Verification items for the finished model (mm, model axes). A direction names the side the tool comes from. Round coordinates to 2 decimals unless told otherwise and drop trailing zeros. Order: outer loops, then holes, each group sorted by start corner. A loop starts at its lowest first (then second) coordinate and runs counter-clockwise, first axis right, second up.
```python
from build123d import *

# Parameters (mm, degrees)
SKETCH_1_R          = 1.95
EXTRUDE_1_DEPTH     = 3
SKETCH_2_R          = 1.45
SKETCH_2_W          = 20
SKETCH_2_H          = 40
CUT_EXTRUDE_1_DEPTH = 10
FILLET_1_R          = 1.5
FILLET_2_R          = 10
FILLET_3_R          = 2


with BuildPart() as part:
    # 草图1 → 凸台-拉伸1 (new body)
    with BuildSketch(Plane.XY):
        Polygon((0, 0), (0, 66), (38, 66), (38, 0), (25, -45.927575687), (25, -78.1), (13, -78.1), (13, -45.927575687), align=None)
        with Locations((4, 40)):
            Circle(SKETCH_1_R, mode=Mode.SUBTRACT)
        with Locations((34, 40)):
            Circle(SKETCH_1_R, mode=Mode.SUBTRACT)
        with Locations((4, 61)):
            Circle(SKETCH_1_R, mode=Mode.SUBTRACT)
        with Locations((34, 61)):
            Circle(SKETCH_1_R, mode=Mode.SUBTRACT)
        with Locations((19, -56.8)):
            Circle(SKETCH_1_R, mode=Mode.SUBTRACT)
        with Locations((19, -69.2)):
            Circle(SKETCH_1_R, mode=Mode.SUBTRACT)
    extrude(amount=EXTRUDE_1_DEPTH)

    # 草图2 → 切除-拉伸1 (cut)
    with BuildSketch(Plane.XY.offset(3)):
        with Locations((12, 15)):
            Circle(SKETCH_2_R)
        with Locations((26, 15)):
            Circle(SKETCH_2_R)
        Polygon((5, 10), (16, 10), (16, -38.16779197), (5, 0.694002842), align=None)
        with Locations((19, 40)):
            Rectangle(SKETCH_2_W, SKETCH_2_H)
        Polygon((22, 10), (22, -38.16779197), (33, 0.694002842), (33, 10), align=None)
    extrude(amount=-CUT_EXTRUDE_1_DEPTH, mode=Mode.SUBTRACT)

    # 圆角1
    fillet_1_edges = [part.edges().sort_by_distance(p)[0] for p in [
        (0, 0, 1.5),
        (38, 0, 1.5),
        (25, -78.1, 1.5),
        (13, -78.1, 1.5),
    ]]
    fillet(fillet_1_edges, radius=FILLET_1_R)

    # 圆角2
    fillet_2_edges = [part.edges().sort_by_distance(p)[0] for p in [
        (25, -45.927575687, 1.5),
        (13, -45.927575687, 1.5),
    ]]
    fillet(fillet_2_edges, radius=FILLET_2_R)

    # 圆角3
    fillet_3_edges = [part.edges().sort_by_distance(p)[0] for p in [
        (0, 66, 1.5),
        (38, 66, 1.5),
        (9, 20, 1.5),
        (9, 60, 1.5),
        (29, 60, 1.5),
        (29, 20, 1.5),
        (5, 0.694002842, 1.5),
        (5, 10, 1.5),
        (16, 10, 1.5),
        (16, -38.16779197, 1.5),
        (22, 10, 1.5),
        (33, 10, 1.5),
        (33, 0.694002842, 1.5),
        (22, -38.16779197, 1.5),
    ]]
    fillet(fillet_3_edges, radius=FILLET_3_R)


solid = part.part
```
1) Draft check along Z on faces 1 (the flat face through (19, -5, 0)), 2 (the flat face through (28, 10, 2)). Enter one of: released by +Z, released by -Z, zero draft, split by the parting line, or undercut.
2) Sectioned sample at A-A on y = 53.5. Record the cut outline in (x, z).
3) Sectioned sample at D-D on z = 0.8. Count the separate pieces of the cut face and the enclosed holes in it, then the cut area to 3 significant figures.
4) Scan lines: probe 1 along X at (y, z) = (0.5, 0.75); probe 2 along X at (y, z) = (43.5, 1); probe 3 along Y at (x, z) = (15, 1.65). Record each from-to range of solid material in increasing order.
5) Go/stop test with flat-tipped pins: pin 1 Ø1.5 at (y, z) = (-5, 1.5) entering from +X; pin 2 Ø2.5 at (x, y) = (4, 61) entering from -Z; pin 3 Ø0.9 at (y, z) = (-8.5, 2) entering from -X. Record where each tip stops, or that it passes through.
6) Tool access check on faces 3 (the flat face through (16, -8, 2)), 4 (the flat face through (25, -62, 1)), 5 (the flat face through (13, -62, 1)), 6 (the flat face through (38, 33, 1)). Record the directions out of +Z, -Z, +X, -X, +Y, -Y that give a thin tool (end or side, any length) a straight path to the whole face; none if there is none.
7) Sectioned sample at C-C on y = -15.5. Record the cut outline in (x, z).
8) Sectioned sample at B-B on x = 19. Record the cut outline in (y, z), then the cut area to 3 significant figures.
Returned:
1. face 1: released by -Z
1. face 2: zero draft
2. outline: (0, 0) - (9, 0) - (9, 3) - (0, 3) - close; (29, 0) - (38, 0) - (38, 3) - (29, 3) - close
3. separate pieces: 1
3. enclosed holes: 11
3. area: 2,580 mm2
4. probe 1: x = 0 to 5.06, 16 to 22, 32.94 to 38
4. probe 2: x = 0 to 9, 29 to 38
4. probe 3: y = -78.1 to -25.49, 9.73 to 20, 60 to 66
5. pin 1: stops at x = 36.8
5. pin 2: passes through
5. pin 3: stops at x = 2.28
6. face 3: +Z, -Z
6. face 4: +Z, -Z, +X, -Y
6. face 5: +Z, -Z, -X, -Y
6. face 6: +Z, -Z, +X, +Y, -Y
7. outline: (4.39, 0) - (9.58, 0) - (9.58, 3) - (4.39, 3) - close; (16, 0) - (22, 0) - (22, 3) - (16, 3) - close; (28.42, 0) - (33.61, 0) - (33.61, 3) - (28.42, 3) - close
8. outline: (-78.1, 0) - (-71.15, 0) - (-71.15, 3) - (-78.1, 3) - close; (-67.25, 0) - (-58.75, 0) - (-58.75, 3) - (-67.25, 3) - close; (-54.85, 0) - (20, 0) - (20, 3) - (-54.85, 3) - close; (60, 0) - (66, 0) - (66, 3) - (60, 3) - close
8. area: 289 mm2
